from build123d import *

# Parameters (mm, degrees)
ESQUISSE1_W                              = 130
ESQUISSE1_H                              = 30
BOSS_EXTRU_1_DEPTH                       = 70
ENL_VEMENT_DE_MATI_RE_R_VOLUTION47_ANGLE = 180
ENL_VEMENT_START                         = -55.237277286
ENL_VEMENT_DE_MATI_RE_R_VOLUTION48_DEPTH = 26.619101243
CONG_1_R                                 = 18
ESQUISSE10_W                             = 19.973037842
ESQUISSE10_H                             = 30
ENL_V_MAT_EXTRU_2_DEPTH                  = 97.695398184
ENL_V_MAT_EXTRU_5_DEPTH                  = 5
ESQUISSE15_R                             = 1.7
ENL_V_MAT_EXTRU_7_DEPTH                  = 101.124922107


# Read off the part's stored shape, not the designer's step: Enlèvement de matière-Révolution48
with BuildPart() as part:
    # Esquisse1 → Boss.-Extru.1 (new body)
    with BuildSketch(Plane.XY):
        Rectangle(ESQUISSE1_W, ESQUISSE1_H)
    extrude(amount=BOSS_EXTRU_1_DEPTH)

    # Esquisse6 → Enlèvement de matière-Révolution47 (revolve, cut)
    with BuildSketch(Plane(origin=(0, 15, 0), x_dir=(1, 0, 0), z_dir=(0, 1, 0))):
        with BuildLine():
            Line((-30, -35), (30, -35))
            add(Edge.make_bspline(
                [(30, -35), (30, -10), (0, -10), (-30, -10), (-30, -35)],
                knots=[0, 0, 0, 1.570796327, 1.570796327, 3.141592654, 3.141592654, 3.141592654], degree=2, weights=[1, 0.707106781, 1, 0.707106781, 1]))
        make_face()
    revolve(axis=Axis((65, 15, 35), (-1, 0, 0)), revolution_arc=ENL_VEMENT_DE_MATI_RE_R_VOLUTION47_ANGLE, mode=Mode.SUBTRACT)

    # Enlèvement de matière-Révolution48 outli → Enlèvement de matière-Révolution48 (cut)
    with BuildSketch(Plane.YZ.offset(ENL_VEMENT_START)):
        with BuildLine():
            Line((15, 27.5), (15, 42.5))
            ThreePointArc((15, 42.5), (7.5, 35), (15, 27.5))
        make_face()
    extrude(amount=ENL_VEMENT_DE_MATI_RE_R_VOLUTION48_DEPTH, mode=Mode.SUBTRACT)

    # Congé1
    cong_1_edges = [part.edges().sort_by_distance(p)[0] for p in [
        (-28.618176043, 7.5, 35),
    ]]
    fillet(cong_1_edges, radius=CONG_1_R)

    # Esquisse10 → Enlèv. mat.-Extru.2 (cut, through all)
    with BuildSketch(Plane(origin=(0, 0, 0), x_dir=(-1, 0, 0), z_dir=(0, 0, -1))):
        with Locations((-55.013481079, 0)):
            Rectangle(ESQUISSE10_W, ESQUISSE10_H)
    extrude(amount=-ENL_V_MAT_EXTRU_2_DEPTH, mode=Mode.SUBTRACT)

    # Esquisse14 → Enlèv. mat.-Extru.5 (cut)
    with BuildSketch(Plane(origin=(0, 15, 0), x_dir=(1, 0, 0), z_dir=(0, 1, 0))):
        with BuildLine():
            Line((-36.95065792, -22.593731953), (-33.568216071, -22.593731953))
            add(Edge.make_bspline(
                [(-32.969763, -47.992109896), (-11.968044376, -80.456384186), (23.634832969, -57.413436774), (59.237710315, -34.370489362), (22.565908506, -12.048229698), (-14.105893303, 10.274029966), (-33.568216071, -22.593731953)],
                knots=[3.621962513, 3.621962513, 3.621962513, 5.414642661, 5.414642661, 7.207322809, 7.207322809, 9.000002957, 9.000002957, 9.000002957], degree=2, weights=[1, 0.624472717, 1, 0.624472717, 1, 0.624472717, 1]))
            Line((-32.969763, -47.992109896), (-36.439122288, -47.992109896))
            add(Edge.make_bspline(
                [(-36.439122288, -47.992109896), (-35.734455038, -49.237206185), (-34.899635372, -50.4303054)],
                knots=[3.575076272, 3.575076272, 3.575076272, 3.671550289, 3.671550289, 3.671550289], degree=2, weights=[1, 0.979509213, 0.961188751]))
            add(Edge.make_bspline(
                [(-34.899635372, -50.4303054), (-11.819428822, -83.415843998), (25.026969924, -59.963213412), (65.234193612, -34.371427073), (24.010934913, -9.515816182), (-13.543091018, 13.127426623), (-35.401513383, -19.963295045)],
                knots=[3.671550289, 3.671550289, 3.671550289, 5.396765185, 5.396765185, 7.218454098, 7.218454098, 8.937188842, 8.937188842, 8.937188842], degree=2, weights=[0.961188751, 0.633569616, 1, 0.613078829, 1, 0.634945981, 0.958737375]))
            add(Edge.make_bspline(
                [(-35.401513383, -19.963295045), (-36.251462308, -21.250003794), (-36.95065792, -22.593731953)],
                knots=[8.937188842, 8.937188842, 8.937188842, 9.04014301, 9.04014301, 9.04014301], degree=2, weights=[0.958737375, 0.978132848, 1]))
        make_face()
        with BuildLine():
            Line((-59.600015614, -22.593731953), (-36.95065792, -22.593731953))
            add(Edge.make_bspline(
                [(-35.401513383, -19.963295045), (-36.251462308, -21.250003794), (-36.95065792, -22.593731953)],
                knots=[8.937188842, 8.937188842, 8.937188842, 9.04014301, 9.04014301, 9.04014301], degree=2, weights=[0.958737375, 0.978132848, 1]))
            Line((-35.401513383, -19.963295045), (-62.094279206, -19.963295045))
            Line((-62.094279206, -19.963295045), (-62.094279206, -50.4303054))
            Line((-62.094279206, -50.4303054), (-34.899635372, -50.4303054))
            add(Edge.make_bspline(
                [(-36.439122288, -47.992109896), (-35.734455038, -49.237206185), (-34.899635372, -50.4303054)],
                knots=[3.575076272, 3.575076272, 3.575076272, 3.671550289, 3.671550289, 3.671550289], degree=2, weights=[1, 0.979509213, 0.961188751]))
            Line((-36.439122288, -47.992109896), (-59.600015614, -47.992109896))
            Line((-59.600015614, -47.992109896), (-59.600015614, -22.593731953))
        make_face()
    extrude(amount=-ENL_V_MAT_EXTRU_5_DEPTH, mode=Mode.SUBTRACT)

    # Esquisse15 → Enlèv. mat.-Extru.7 (cut, through all)
    with BuildSketch(Plane(origin=(0, 15, 0), x_dir=(1, 0, 0), z_dir=(0, 1, 0))):
        with Locations(Location((35, -7.5, 0), (0, 0, 270))):
            Circle(ESQUISSE15_R)
        with Locations(Location((35, -62.5, 0), (0, 0, 270))):
            Circle(ESQUISSE15_R)
        with Locations(Location((-35, -62.5, 0), (0, 0, 270))):
            Circle(ESQUISSE15_R)
        with Locations(Location((-35, -7.5, 0), (0, 0, 270))):
            Circle(ESQUISSE15_R)
    extrude(amount=-ENL_V_MAT_EXTRU_7_DEPTH, mode=Mode.SUBTRACT)


solid = part.part
The listing builds one solid part. Answer for the finished solid, in the listing's coordinates (mm). A direction names the side the tool comes from. Coordinates: 2 decimals unless noted, no trailing zeros. Loops run counter-clockwise (first coordinate to the right, second up) from the corner with the lowest first, then second, coordinate; pieces in that order, holes last. Notation, with made-up numbers: M -1,-39 L 5,-39 A21 ccw 5,-11 Z; hole C 27,63 d10. An arc over 180 degrees is marked long. Answer in a Markdown table with one row per item.
1) Find section A-A (x = -46). Determine the outline of the cut face in (y, z).
Answers below:
| item | result |
|---|---|
| outline | M -15,0 L 15,0 L 15,19.96 L 10,19.96 L 10,22.59 L 15,22.59 L 15,27.5 A7.5 cw 15,42.5 L 15,47.99 L 10,47.99 L 10,50.43 L 15,50.43 L 15,70 L -15,70 Z |
2) Given pin 1 (2 mm diameter, centred on x = -35, z = 7.5, fed in from +Y); pin 2 (4 mm diameter, centred on x = -35, z = 62.5, fed in from -Y), each flat-ended and moving along its own axis, determine where each tip first touches the part or whether it passes through.
Answers below:
| item | result |
|---|---|
| pin 1 | through |
| pin 2 | y = -15 |
3) Which of the six approach directions +Z, -Z, +X, -X, +Y, -Y give full straight-line access (tool end or side, diameter ignored) to faces 5 (the cylindrical face through (-47.09, 7.5, 35.16)), 6 (the cylindrical face through (-36.03, 0.21, 61.15))?
Answers below:
| item | result |
|---|---|
| face 5 | +Y |
| face 6 | +Y, -Y |
4) Determine the mould class of faces 1 (the flat face through (-65, 0, 35)), 2 (the flat face through (-47, 13, 22.594)), 3 (the cylindrical face through (-36.66, 0.21, 7.13)), 4 (the flat face through (-11, 0, 0)) for opening direction Z: released by +Z, released by -Z, zero draft, split by the parting line, or undercut.
Answers below:
| item | result |
|---|---|
| face 1 | zero draft |
| face 2 | undercut |
| face 3 | undercut |
| face 4 | released by -Z |
5) Find section B-B (y = -5.5). Count the separate pieces of the cut face and the enclosed holes in it, then the cut area to 3 significant figures.
Answers below:
| item | result |
|---|---|
| separate pieces | 1 |
| enclosed holes | 5 |
| area | 6,890 mm^2 |
6) Find the intervals of material crossed by probe 1 along X at (y, z) = (-8, 7.5); probe 2 along X at (y, z) = (6, 7); probe 3 along Y at (x, z) = (1, 5.5), in increasing order.
Answers below:
| item | result |
|---|---|
| probe 1 | -65 to -36.7, -33.3 to 33.3, 36.7 to 45.03 |
| probe 2 | -65 to -36.62, -33.38 to 33.38, 36.62 to 45.03 |
| probe 3 | -15 to 10 |
